For this review, use the dimensioned drawing (mm, ordinates from the lowest corner) and the shaded views. A direction names the side the tool comes from. Round coordinates to 2 decimals unless told otherwise and drop trailing zeros. Loops run counter-clockwise (first coordinate to the right, second up) from the corner with the lowest first, then second, coordinate; pieces in that order, holes last. Notation, with made-up numbers: (76.5, 21) -> (116.5, 21) arc R18 ccw to (116.5, 28) -> close; hole circle Ø10 at (19.5, 78). An arc over 180 degrees is marked (long way). Write each question's results on one line, items separated by ' | '.
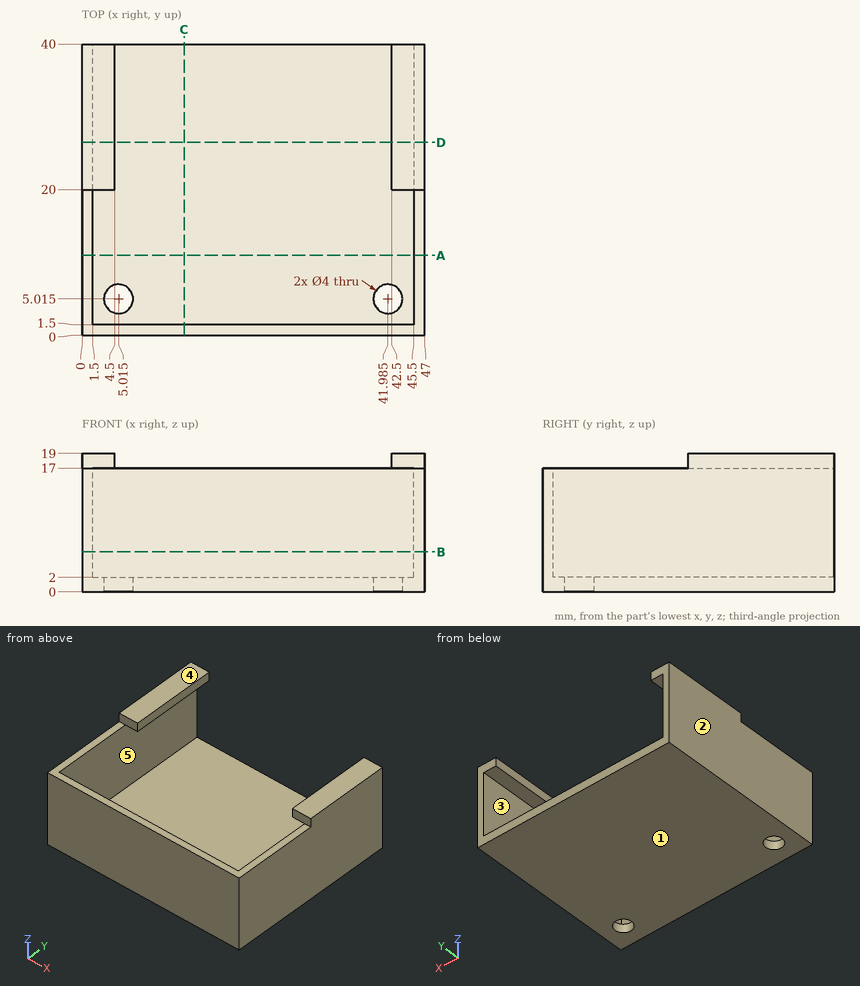
1. Consider section B-B (z = 5.5). State the section outline as (x, y) points.
Values found:
outline: (0, 0) -> (47, 0) -> (47, 40) -> (45.5, 40) -> (45.5, 1.5) -> (1.5, 1.5) -> (1.5, 40) -> (0, 40) -> close
2. To check wall thickness, follow probe 1 along X at (y, z) = (32, 13.75); probe 2 along Z at (x, y) = (3, 23); probe 3 along Z at (x, y) = (36.5, 10). State the ranges of each line that lie inside material, in increasing order.
Values found:
probe 1: x = 0 to 1.5, 45.5 to 47 | probe 2: z = 0 to 2, 17 to 19 | probe 3: z = 0 to 2
3. Consider section D-D (y = 26.5). State the section outline as (x, z) points, plus the area to 3 significant figures.
Values found:
outline: (0, 0) -> (47, 0) -> (47, 19) -> (42.5, 19) -> (42.5, 17) -> (45.5, 17) -> (45.5, 2) -> (1.5, 2) -> (1.5, 17) -> (4.5, 17) -> (4.5, 19) -> (0, 19) -> close | area: 157 mm2
4. Tool access review of the marked faces 4 and 5: name each direction out of +Z, -Z, +X, -X, +Y, -Y from which nothing blocks a thin tool from reaching the whole face with its end or side.
Values found:
face 4: +Z, +X, -X, +Y, -Y | face 5: +Y
5. Draft analysis for pull direction Z (two halves, no side actions). For the marked faces 1, 2 and 3, state which applies: released by +Z, released by -Z, zero draft, split by the parting line, or undercut.
Values found:
face 1: released by -Z | face 2: zero draft | face 3: undercut
6. For pin 1 (2.5 mm diameter, centred on x = 41.99, y = 5.01, fed in from +Z); pin 2 (2 mm diameter, centred on x = 30.5, z = 10.5, fed in from +Y); pin 3 (10 mm diameter, centred on x = 25, y = 8.5, fed in from +Z), all flat-tipped, find the tip position at first contact; note any pin that passes through.
Values found:
pin 1: passes through | pin 2: stops at y = 1.5 | pin 3: stops at z = 2
7. Consider section C-C (x = 14). State the section outline as (y, z) points.
Values found:
outline: (0, 0) -> (40, 0) -> (40, 2) -> (1.5, 2) -> (1.5, 17) -> (0, 17) -> close
8. Consider section A-A (y = 11). State the section outline as (x, z) points.
Values found:
outline: (0, 0) -> (47, 0) -> (47, 17) -> (45.5, 17) -> (45.5, 2) -> (1.5, 2) -> (1.5, 17) -> (0, 17) -> close
